Design review of the part shown in the three views and the two pictorial views. Dimensions are in mm from the part's minimum x, y and z. A direction names the side the tool comes from. Coordinates: 2 decimals unless noted, no trailing zeros. Write each loop counter-clockwise with the first axis right and the second up, starting at its lowest first coordinate (ties: lowest second). Pieces come first, ordered by that corner, then holes. Notation, with made-up numbers: (20.5, 16) - (32.5, 16) arc R14 cw to (32.5, 35) - close; hole circle Ø9 at (-13, 79). An arc over 180 degrees is marked (long way). Write each question's results on one line, items separated by ' | '.
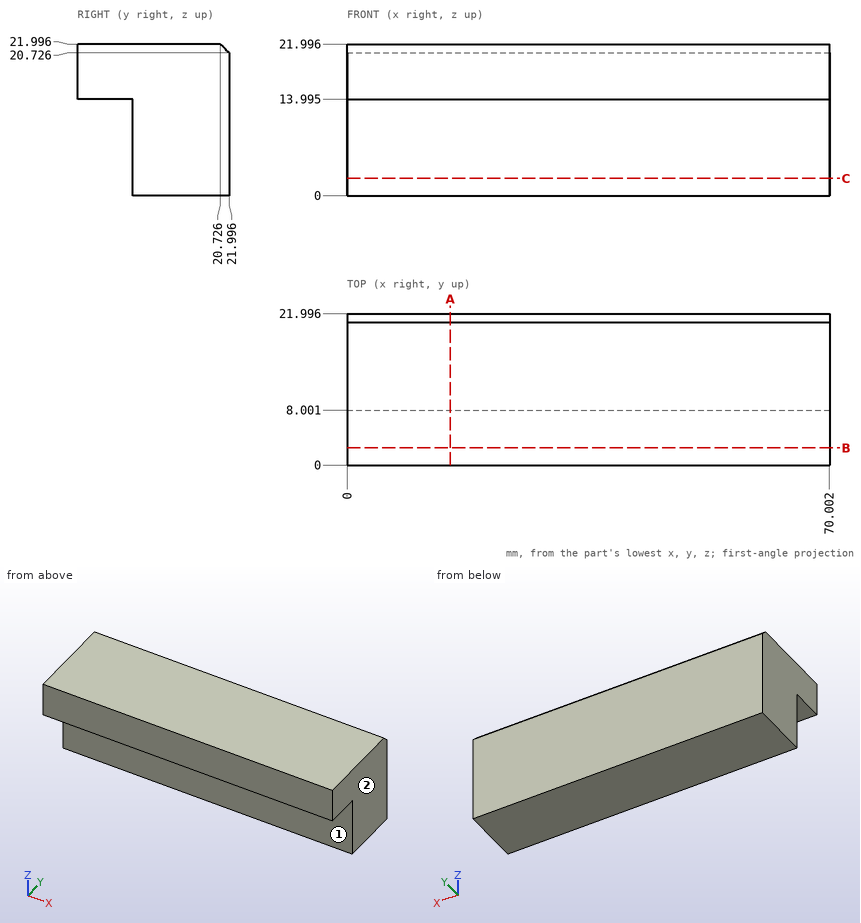
Q1. Wall thickness on line 1 along Z through (x, y) = (47.5, 3.75) (1 decimal); line 2 along Y through (x, z) = (53, 11.25); line 3 along Z through (x, y) = (30, 21) (1 decimal): over which ranges is each line inside the solid? List them lowest first. Write a range as from..to.
Results found:
line 1: 14..22 | line 2: 8..22 | line 3: 0..21.7
Q2. Take a section at B-B on y = 2.5. State the section outline as (x, z) points (1 decimal).
Results found:
outline: (0, 14) - (70, 14) - (70, 22) - (0, 22) - close
Q3. For pin 1 (4 mm diameter, centred on x = 23.5, z = 8.5, fed in from -Y); pin 2 (4 mm diameter, centred on x = 48, y = 5, fed in from -Z) (1 decimal), all flat-tipped, find the tip position at first contact; note any pin that passes through.
Results found:
pin 1: y = 8 | pin 2: z = 14
Q4. For the marked faces 1 and 2, list the 3-axis set-ups (+Z, -Z, +X, -X, +Y, -Y) from which the entire face can be reached by the end or side of a thin tool; tool diameter is ignored.
Results found:
face 1: -Z, +X, -X, -Y | face 2: +Z, -Z, +X, +Y, -Y
Q5. Take a section at C-C on z = 2.5. State the section outline as (x, y) points.
Results found:
outline: (0, 8) - (70, 8) - (70, 22) - (0, 22) - close
Q6. Take a section at A-A on x = 15. State the section outline as (y, z) points (1 decimal), plus the area to 3 significant figures.
Results found:
outline: (0, 14) - (8, 14) - (8, 0) - (22, 0) - (22, 20.7) - (20.7, 22) - (0, 22) - close | area: 371 mm2
